from build123d import *

# Parameters (mm, degrees)
F0_W     = 70
F0_H     = 70
F1_DEPTH = 110
F1_TAPER = 10
F2_R     = 10
F3_T     = -2


with BuildPart() as f1:
    # F0 (on Top) → F1 (new body)
    with BuildSketch(Plane.XY):
        Rectangle(F0_W, F0_H)
    extrude(amount=F1_DEPTH, taper=F1_TAPER)

    # F2
    f2_edges = [f1.edges().sort_by_distance(p)[0] for p in [
        (25.302016, -25.302016, 55),
        (25.302016, 25.302016, 55),
        (-25.302016, -25.302016, 55),
        (-25.302016, 25.302016, 55),
    ]]
    fillet(f2_edges, radius=F2_R)

    # F3
    f3_openings = [f1.faces().sort_by_distance(p)[0] for p in [
        (0, 0, 0),
        (0, 0, 110),
    ]]
    offset(amount=F3_T, openings=f3_openings)


solid = f1.part
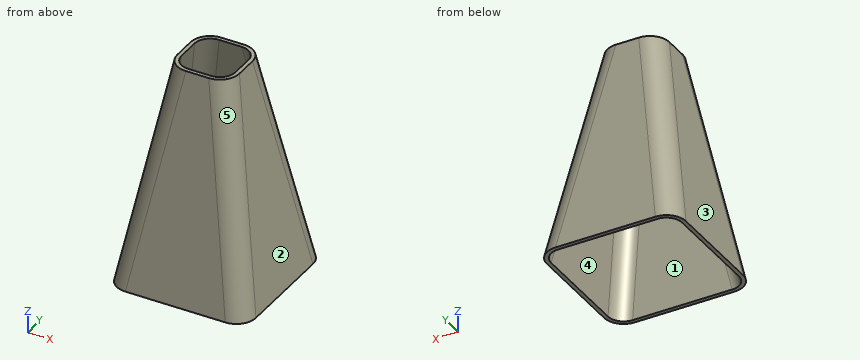
The model under review builds one solid part; all positions refer to its coordinate system, in mm. Face numbers are marked on the shaded views. A direction names the side the tool comes from. Round coordinates to 2 decimals unless told otherwise and drop trailing zeros. Order: outer loops, then holes, each group sorted by start corner. A loop starts at its lowest first (then second) coordinate and runs counter-clockwise, first axis right, second up. Notation, with made-up numbers: (16, 30.5) -> (69, 30.5) arc R21 cw to (69, 64.5) -> close; hole circle Ø8 at (13.25, 57.5). An arc over 180 degrees is marked (long way). Write item = value, one per line. Start each with the question number.
Item 1: For the marked faces 1 and 2, list the 3-axis set-ups (+Z, -Z, +X, -X, +Y, -Y) from which the entire face can be reached by the end or side of a thin tool; tool diameter is ignored.
Item 2: Clearance check with flat-ended pins moving along their axes: pin 1 Ø1.5 at (y, z) = (17, 29.5) entering from -X; pin 2 Ø1.5 at (x, z) = (13, 60.5) entering from -Y; pin 3 Ø12 at (x, z) = (10.5, 69) entering from -Y; pin 4 Ø4 at (x, y) = (6.5, -13) entering from +Z. State where each tip first meets the part, or that it passes through.
Item 3: Consider section A-A on y = -1. Write out the cut boundary in (x, z), plus the area to 3 significant figures.
Item 4: For line 1 along Y through (x, z) = (-15, 68.5); line 2 along X through (y, z) = (-3.5, 45); line 3 along X through (y, z) = (-16, 63.5), list the stretches that pass through material, from the lowest coordinate up.
Item 5: Mouldability with a two-part tool opening along X and no side actions: class the marked faces 3, 4 and 5 as released by +X, released by -X, zero draft, split by the parting line, or undercut.
Conclusion:
q1.face_1 = -Z
q1.face_2 = +Z, +X, +Y, -Y
q2.pin_1 = -29.93
q2.pin_2 = -24.46
q2.pin_3 = -23.89
q2.pin_4 = 110
q3.outline = (-35, 0) -> (-32.97, 0) -> (-13.57, 110) -> (-15.6, 110) -> close; (13.57, 110) -> (32.97, 0) -> (35, 0) -> (15.6, 110) -> close
q3.area = 447 mm2
q4.line_1 = -22.74 to -20.64, 20.64 to 22.74
q4.line_2 = -27.07 to -25.03, 25.03 to 27.07
q4.line_3 = -23.59 to -21.49, 21.49 to 23.59
q5.face_3 = released by -X
q5.face_4 = undercut
q5.face_5 = released by +X
